from build123d import *


with BuildPart() as part:
    # Sketch1 → Revolve1 (revolve)
    with BuildSketch(Plane.XY, mode=Mode.PRIVATE) as revolve1_sk:
        with BuildLine():
            Line((-7.9375, 0), (-7.9375, 150.8125))
            Line((-7.9375, 150.8125), (-8.6995, 150.8125))
            ThreePointArc((-8.6995, 150.8125), (-9.283216648, 151.054283352), (-9.525, 151.638))
            Line((-9.525, 151.638), (-9.525, 152.4))
            Line((-9.525, 152.4), (-11.1125, 152.4))
            Line((-11.1125, 152.4), (-9.525, 149.225))
            Line((-9.525, 149.225), (-9.525, 7.14375))
            ThreePointArc((-9.525, 7.14375), (-9.757483992, 6.582483992), (-10.31875, 6.35))
            Line((-10.31875, 6.35), (-11.1125, 6.35))
            ThreePointArc((-11.1125, 6.35), (-11.90625, 5.55625), (-11.1125, 4.7625))
            Line((-11.1125, 4.7625), (-10.31875, 4.7625))
            ThreePointArc((-10.31875, 4.7625), (-9.757483992, 4.530016008), (-9.525, 3.96875))
            Line((-9.525, 3.96875), (-9.525, 0))
            Line((-9.525, 0), (-7.9375, 0))
        make_face()
    revolve(revolve1_sk.sketch.rotate(Axis((0, 0, 0), (0, 1, 0)), 270), axis=Axis((0, 0, 0), (0, 1, 0)))


solid = part.part
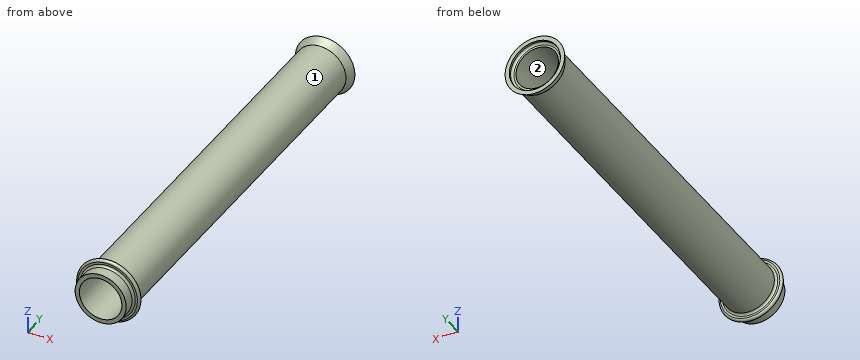
Part model, mm, in its own coordinate system. Face numbers are marked on the shaded views. Coordinates: 2 decimals unless noted, no trailing zeros. Use a Markdown table: item, result. Add a question column.
Item 1: Probe probe 1 along X at (y, z) = (94.5, -0.25); probe 2 along X at (y, z) = (72, 5.75); probe 3 along Y at (x, z) = (7.25, -8.25). List the from-to ranges inside material, lowest first.
Item 2: Pull direction X, two halves, no side cores. Call the marked faces 1 and 2: +X half, -X half, draft (parallel to the pull), parting line (faces both ways), or undercut.
Item 3: Flat gauge pins, fed straight in: P1, Ø3, axis at x = 3.5, y = 54.5, coming from the +Z side; P2, Ø1.5, axis at x = -9, y = 33.5, coming from the -Z side; P3, Ø12, axis at x = 9, y = 16.5, coming from the -Z side. Where does each tip first touch, or does it go through?
Geometry says:
| question | item | result |
|---|---|---|
| 1 | probe 1 | -9.52 to -7.93, 7.93 to 9.52 |
| 1 | probe 2 | -7.59 to -5.47, 5.47 to 7.59 |
| 1 | probe 3 | 4.76 to 6.35, 152.14 to 152.4 |
| 2 | face 1 | parting line |
| 2 | face 2 | undercut |
| 3 | P1 | z = 9.31 |
| 3 | P2 | z = -4.76 |
| 3 | P3 | z = -9.04 |
